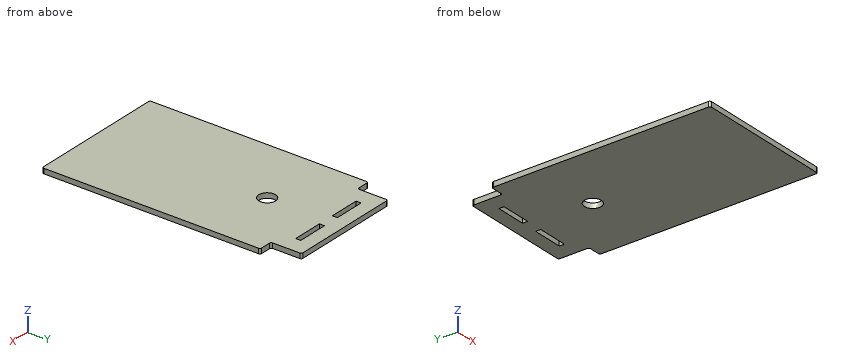
```python
from build123d import *

# Parameters (mm, degrees)
MODEL_R                 = 5
MODEL_W                 = 18.163611367
MODEL_H                 = 3
MODEL_W_2               = 18.163611368
SALIENTE_EXTRUIR1_DEPTH = 3


with BuildPart() as part:
    # Model → Saliente-Extruir1 (new body)
    with BuildSketch(Plane.XY):
        with BuildLine():
            Line((95.99768192, -24.017865973), (95.99768192, 103.764725177))
            ThreePointArc((95.99768192, 103.764725177), (95.708514347, 104.473363697), (95.002958892, 104.769974448))
            Line((95.002958892, 104.769974448), (88.830267122, 104.802462525))
            ThreePointArc((88.830267122, 104.802462525), (88.124711667, 105.099073276), (87.835544094, 105.807711796))
            Line((87.835544094, 105.807711796), (87.824904655, 121.982134027))
            ThreePointArc((87.824904655, 121.982134027), (87.532011436, 122.689240808), (86.824904655, 122.982134027))
            Line((86.824904655, 122.982134027), (22.49768192, 122.982134027))
            ThreePointArc((22.49768192, 122.982134027), (21.790575139, 122.689240808), (21.49768192, 121.982134027))
            Line((21.49768192, 121.982134027), (21.49768192, 105.982134027))
            ThreePointArc((21.49768192, 105.982134027), (21.204788701, 105.275027246), (20.49768192, 104.982134027))
            Line((20.49768192, 104.982134027), (14.324904655, 104.982134027))
            ThreePointArc((14.324904655, 104.982134027), (13.617797874, 104.689240808), (13.324904655, 103.982134027))
            Line((13.324904655, 103.982134027), (13.324904655, 59.982134027))
            Line((13.324904655, 59.982134027), (13.324904655, 53.982134027))
            Line((13.324904655, 53.982134027), (13.324904655, 21.297944303))
            Line((13.324904655, 21.297944303), (13.324904655, -24.017865973))
            ThreePointArc((13.324904655, -24.017865973), (13.617797874, -24.724972754), (14.324904655, -25.017865973))
            Line((14.324904655, -25.017865973), (94.99768192, -25.017865973))
            ThreePointArc((94.99768192, -25.017865973), (95.704788701, -24.724972754), (95.99768192, -24.017865973))
        make_face()
        with Locations((54.561293288, 76.782134027)):
            Circle(MODEL_R, mode=Mode.SUBTRACT)
        with Locations((68.743098972, 113.282134027)):
            Rectangle(MODEL_W, MODEL_H, mode=Mode.SUBTRACT)
        with Locations((40.579487604, 113.282134027)):
            Rectangle(MODEL_W_2, MODEL_H, mode=Mode.SUBTRACT)
    extrude(amount=SALIENTE_EXTRUIR1_DEPTH)


solid = part.part
```
Read the model definition and answer for the solid it produces. Units are mm, in the model's axes. Coordinates: 2 decimals unless noted, no trailing zeros. Write each loop counter-clockwise with the first axis right and the second up, starting at its lowest first coordinate (ties: lowest second). Pieces come first, ordered by that corner, then holes. Notation, with made-up numbers: (-40, -25) -> (-5, -25) arc R17 cw to (-5, 3) -> close; hole circle Ø2 at (31.25, 32.25). An arc over 180 degrees is marked (long way). Answer as a JSON object with one key per item and string values.
Q1. The part is cut by section B-B on z = 0.8. Give the vertices of the cut face in (x, y), then the cut area to 3 significant figures.
The answers:
{"outline": "(13.32, -24.02) arc R1 ccw to (14.32, -25.02) -> (95, -25.02) arc R1 ccw to (96, -24.02) -> (96, 103.76) arc R1 ccw to (95, 104.77) -> (88.83, 104.8) arc R1 cw to (87.84, 105.81) -> (87.82, 121.98) arc R1 ccw to (86.82, 122.98) -> (22.5, 122.98) arc R1 ccw to (21.5, 121.98) -> (21.5, 105.98) arc R1 cw to (20.5, 104.98) -> (14.32, 104.98) arc R1 ccw to (13.32, 103.98) -> close; hole (31.5, 111.78) -> (49.66, 111.78) -> (49.66, 114.78) -> (31.5, 114.78) -> close; hole circle Ø10 at (54.56, 76.78); hole (59.66, 111.78) -> (77.82, 111.78) -> (77.82, 114.78) -> (59.66, 114.78) -> close", "area": "11,800 mm2"}
Q2. The part is cut by section A-A on x = 61.5. Give the vertices of the cut face in (y, z).
The answers:
{"outline": "(-25.02, 0) -> (111.78, 0) -> (111.78, 3) -> (-25.02, 3) -> close; (114.78, 0) -> (122.98, 0) -> (122.98, 3) -> (114.78, 3) -> close"}
Q3. Consider line 1 (X direction, y = 113.5, z = 2.95); line 2 (Y direction, x = 38, z = 1.25); line 3 (Y direction, x = 17, z = 0.85). Determine where each line is inside the solid, lowest interval first. Write a range as [from, to].
The answers:
{"line 1": "x = [21.5, 31.5], [49.66, 59.66], [77.82, 87.83]", "line 2": "y = [-25.02, 111.78], [114.78, 122.98]", "line 3": "y = [-25.02, 104.98]"}
Q4. Flat-ended cylindrical pins translate along their axes: pin 1 Ø0.9 at (x, z) = (17.5, 1) entering from +Y; pin 2 Ø10 at (x, y) = (31, 101) entering from -Z; pin 3 Ø9 at (x, y) = (54.56, 76.78) entering from +Z; pin 4 Ø0.9 at (y, z) = (112.5, 1.5) entering from +X. Find the tip coordinate at first contact, or state that the pin passes through.
The answers:
{"pin 1": "stops at y = 104.98", "pin 2": "stops at z = 0", "pin 3": "passes through", "pin 4": "stops at x = 87.83"}
